Geometry check sheet. Reference: the model listing, model coordinates, mm. A direction names the side the tool comes from. Coordinates: 2 decimals unless noted, no trailing zeros. Write each loop counter-clockwise with the first axis right and the second up, starting at its lowest first coordinate (ties: lowest second). Pieces come first, ordered by that corner, then holes.
from build123d import *

# Parameters (mm, degrees)
PAD_DEPTH       = 4.763
SKETCH001_R     = 2.25
SKETCH001_R_2   = 3
POCKET_DEPTH    = 4.764
FILLET_R        = 5
SKETCH003_R     = 2
POCKET001_DEPTH = 2


with BuildPart() as part:
    # Sketch → Pad (new body)
    with BuildSketch(Plane.XY):
        with BuildLine():
            ThreePointArc((75.749521, 0), (0, 14.9), (-75.749521, 0))
            Line((-104.25, 0), (-75.749521, 0))
            Line((-104.25, 0), (-104.25, 30.01692))
            ThreePointArc((104.25, 30.01692), (0, 55), (-104.25, 30.01692))
            Line((104.25, 30.01692), (104.25, 0))
            Line((75.749521, 0), (104.25, 0))
        make_face()
    extrude(amount=PAD_DEPTH)

    # Sketch001 (on Face8 of Pad) → Pocket (cut, through all)
    with BuildSketch(Plane.XY.offset(4.763)):
        with Locations((-31, 45.5)):
            Circle(SKETCH001_R)
        with Locations((36, 45.5)):
            Circle(SKETCH001_R)
        with Locations((36, 18)):
            Circle(SKETCH001_R)
        with Locations((-31, 18)):
            Circle(SKETCH001_R)
        with Locations((-90, 14.25)):
            Circle(SKETCH001_R_2)
        with Locations((-86, 32.75)):
            Circle(SKETCH001_R_2)
        with Locations((86, 32.75)):
            Circle(SKETCH001_R_2)
        with Locations((90, 14.25)):
            Circle(SKETCH001_R_2)
    extrude(amount=-POCKET_DEPTH, mode=Mode.SUBTRACT)

    # Fillet
    fillet_edges = [part.edges().sort_by_distance(p)[0] for p in [
        (-104.25, 30.01692, 2.3815),
        (-104.25, 0, 2.3815),
        (104.25, 30.01692, 2.3815),
        (-75.749521, 0, 2.3815),
        (75.749521, 0, 2.3815),
        (104.25, 0, 2.3815),
    ]]
    fillet(fillet_edges, radius=FILLET_R)

    # Sketch003 (on Face5 of Fillet) → Pocket001 (cut)
    with BuildSketch(Plane.XY.offset(4.763)):
        with Locations((2.5, 31.75)):
            Circle(SKETCH003_R)
    extrude(amount=-POCKET001_DEPTH, mode=Mode.SUBTRACT)


solid = part.part
1. Sectioned sample at A-A, the plane z = 1.1. Give the number of separate pieces and of enclosed holes in the cut face, and give its area (3 significant figures).
Computed values:
separate pieces: 1
enclosed holes: 8
area: 8,060 mm2
2. Gauge pin test, flat ends, axial feed: pin 1 Ø7 at (x, y) = (-86, 32.75) entering from +Z; pin 2 Ø3 at (x, y) = (2.5, 31.75) entering from +Z. Record the tip position at first contact, or that the pin passes through.
Computed values:
pin 1: stops at z = 4.76
pin 2: stops at z = 2.76
3. Sectioned sample at C-C, the plane x = -31. Record the boundary of the cut face in (y, z).
Computed values:
outline: (12.48, 0) - (15.75, 0) - (15.75, 4.76) - (12.48, 4.76) - close; (20.25, 0) - (43.25, 0) - (43.25, 4.76) - (20.25, 4.76) - close; (47.75, 0) - (52.9, 0) - (52.9, 4.76) - (47.75, 4.76) - close
4. Thickness scan on line 1 along X through (y, z) = (32.5, 3.65); line 2 along Y through (x, z) = (-31, 2.2); line 3 along X through (y, z) = (20, 3.6). Record the ranges inside material, lowest first.
Computed values:
line 1: x = -99.22 to -88.99, -83.01 to 0.65, 4.35 to 83.01, 88.99 to 99.22
line 2: y = 12.48 to 15.75, 20.25 to 43.25, 47.75 to 52.9
line 3: x = -104.25 to -32.03, -29.97 to 34.97, 37.03 to 104.25
5. Sectioned sample at D-D, the plane x = 2.5. Record the boundary of the cut face in (y, z).
Computed values:
outline: (14.88, 0) - (54.99, 0) - (54.99, 4.76) - (33.75, 4.76) - (33.75, 2.76) - (29.75, 2.76) - (29.75, 4.76) - (14.88, 4.76) - close
6. Access from +Z, -Z, +X, -X, +Y, -Y to the whole of each face (thin tool, end or side, straight path). Record for faces 1 (the cylindrical face through (-102.75, 1.43, 2.41)), 2 (the flat face through (2, 32, 2.763)).
Computed values:
face 1: +Z, -Z, -X, -Y
face 2: +Z
7. Sectioned sample at B-B, the plane x = -91. Record the boundary of the cut face in (y, z).
Computed values:
outline: (0, 0) - (11.42, 0) - (11.42, 4.76) - (0, 4.76) - close; (17.08, 0) - (36.23, 0) - (36.23, 4.76) - (17.08, 4.76) - close
8. Draft check along X on faces 3 (the cylindrical face through (103.515, 29.537, 2.415)), 4 (the flat face through (88, 0, 2)), 5 (the cylindrical face through (-103.515, 29.537, 2.415)), 6 (the cylindrical face through (1.074, 14.897, 2.348)). Enter one of: released by +X, released by -X, zero draft, split by the parting line, or undercut.
Computed values:
face 3: released by +X
face 4: zero draft
face 5: released by -X
face 6: undercut
